Check sheet for the modelled part. Datum: model origin and axes. Units: mm. Coordinates: 2 decimals unless noted, no trailing zeros. Loops run counter-clockwise (first coordinate to the right, second up) from the corner with the lowest first, then second, coordinate; pieces in that order, holes last.
```python
from build123d import *

# Parameters (mm, degrees)
SKETCH1_R           = 3
BOSS_EXTRUDE1_DEPTH = 6


with BuildPart() as part:
    # Sketch1 → Boss-Extrude1 (new body)
    with BuildSketch(Plane.XY):
        with BuildLine():
            Line((210, 399.806072497), (-10, 399.806072497))
            Line((-10, 399.806072497), (-10, 396.306072497))
            Line((-10, 396.306072497), (193.636931828, 396.306072497))
            Line((193.636931828, 396.306072497), (210, 384.806072497))
            ThreePointArc((210, 384.806072497), (217.5, 392.306072497), (210, 399.806072497))
        make_face()
        with Locations((210, 392.306072497)):
            Circle(SKETCH1_R, mode=Mode.SUBTRACT)
    extrude(amount=BOSS_EXTRUDE1_DEPTH)


solid = part.part
```
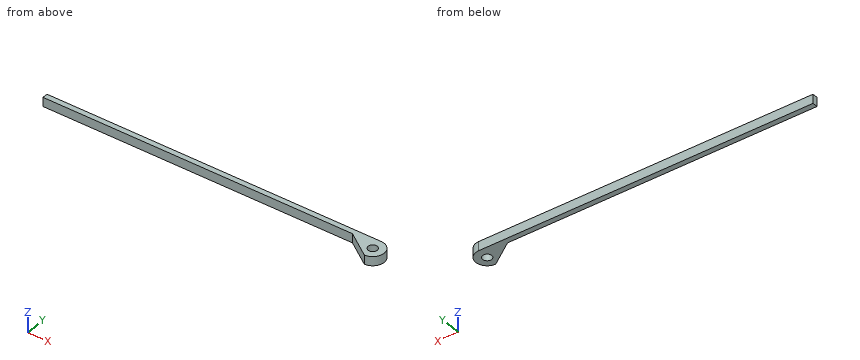
1) Scan lines: line 1 (Y direction, x = 210, z = 4.2); line 2 (X direction, y = 391, z = 3.8); line 3 (X direction, y = 390.75, z = 4.6). Record each from-to range of solid material in increasing order.
Answer sheet:
line 1: y = 384.81 to 389.31, 395.31 to 399.81
line 2: x = 201.19 to 207.3, 212.7 to 217.39
line 3: x = 201.54 to 207.44, 212.56 to 217.34
2) Section check B-B on z = 3.2. Enter the section's corners in (x, y), plus the area to 3 significant figures.
Answer sheet:
outline: (-10, 396.31) - (193.64, 396.31) - (210, 384.81) arc R7.5 ccw to (210, 399.81) - (-10, 399.81) - close; hole circle Ø6 at (210, 392.31)
area: 924 mm2
3) Section check A-A on x = 114. Enter the section's corners in (y, z).
Answer sheet:
outline: (396.31, 0) - (399.81, 0) - (399.81, 6) - (396.31, 6) - close
4) Depth check by flat-ended pin: pin 1 (3 mm diameter, centred on x = 57.5, z = 3, fed in from -Y). Enter the tip coordinate at first touch or a pass-through.
Answer sheet:
pin 1: stops at y = 396.31
